Autodesk Inventor part; units mm, degrees
ref_plane "YZ Plane" through (0, 0, 0) normal (1, 0, 0) x (0, 1, 0)
ref_plane "XZ Plane" through (0, 0, 0) normal (0, 1, 0) x (-1, 0, 0)
ref_plane "XY Plane" through (0, 0, 0) normal (0, 0, 1) x (1, 0, 0)
sketch "Sketch1" plane through (0, 0, 0) normal (0, 0, 1) x (1, 0, 0)
  circle A0 centre (0, 0) radius 20
  circle A1 centre (0, 0) radius 23
  dimension "d0" = 40
  dimension "d1" = 46
extrude "Extrusion1" add sketch "Sketch1" along normal mid plane 330
sketch "Sketch2" plane through (0, 0, 0) normal (1, 0, 0) x (0, 1, 0)
  line L0 (0, 210) -> (0, -210)
  line L1 (-210, 0) -> (210, 0)
  point P0 (0, 0)
  point P1 (0, 110)
  point P2 (0, 0)
  point P3 (0, -110)
  dimension "d4" = 110
  dimension "d5" = 110
hole "Hole1" at (0, 0, 110) at (0, 0, 0) at (0, 0, -110) direction (-1, 0, 0) diameter 4.5 end through all
sketch "Sketch3" plane through (0, 0, 0) normal (1, 0, 0) x (0, 1, 0)
  line L0 (23, -145) -> (7, -145)
  line L1 (7, -145) -> (7, 145)
  line L2 (7, 145) -> (23, 145)
  line L3 (23, 145) -> (23, -145)
  line L4 (23, 165) -> (-23, 165)
  line L5 (-23, -165) -> (23, -165)
  line L6 (0, 297.5) -> (0, -297.5)
  point P0 (0, 0)
  dimension "d13" = 20
  dimension "d14" = 20
  dimension "d15" = 7
extrude "Extrusion2" cut sketch "Sketch3" along normal through all both and the other way through all
fillet "Fillet1" radius 2 4 edges at (20.3219, 7, -145) (-20.3219, 7, -145) (20.3219, 7, 145) (-20.3219, 7, 145)
properties part number "Pancake_Tilt Pipe_3 Lanes" material "PVC-Piping"
Geometry: final body of the model. Coordinates: model frame, mm. A direction names the side the tool comes from. Coordinates: 2 decimals unless noted, no trailing zeros. Order: outer loops, then holes, each group sorted by start corner. A loop starts at its lowest first (then second) coordinate and runs counter-clockwise, first axis right, second up.
Item 1: Contact query for flat-ended pins moving along their axis: P1, Ø10, axis at x = 18, y = -6, coming from the -Z side; P2, Ø2.5, axis at x = 21, z = 0.5, coming from the +Y side; P3, Ø10, axis at y = -12.5, z = 69.5, coming from the +X side; P4, Ø3.5, axis at y = 0, z = 0, coming from the -X side. Output: stop coordinate, or through.
Answer:
P1: stops at z = -165
P2: stops at y = 7
P3: stops at x = 21.74
P4: stops at x = 19.92
Item 2: Section query B-B (z = 17). Output: boundary loops of the cut face in (x, y) (3 decimals).
Answer:
outline: (-21.909, 7) arc R23 ccw (long way) to (21.909, 7) - (18.735, 7) arc R20 cw (long way) to (-18.735, 7) - close
Item 3: Access query for faces 4 (the face through (-4.336, -19.524, 2.31)), 5 (the face through (-1.7, 20.1, 145)). Directions: +Z, -Z, +X, -X, +Y, -Y. A direction counts if a zero-diameter tool reaches every point of the face in a straight line with its end or side. Return the directions, or none.
Answer:
face 4: +Z, -Z
face 5: +X, -X, +Y
Item 4: Section query A-A (x = -9). Output: boundary loops of the cut face in (y, z), then the cut area to 3 significant figures.
Answer:
outline: (-21.17, -165) - (-17.86, -165) - (-17.86, 165) - (-21.17, 165) - close; (17.86, -165) - (21.17, -165) - (21.17, -145) - (17.86, -145) - close; (17.86, 145) - (21.17, 145) - (21.17, 165) - (17.86, 165) - close
area: 1,220 mm2
Item 5: Material intervals for line 1 along Z through (x, y) = (18, 13.5); line 2 along X through (y, z) = (0, -29); line 3 along X through (y, z) = (-16, 117), sorted ascending.
Answer:
line 1: z = -165 to -145, 145 to 165
line 2: x = -23 to -20, 20 to 23
line 3: x = -16.52 to -12, 12 to 16.52
Item 6: Draft query along Z for faces 1 (the face through (-1.7, 20.2, -145)), 2 (the face through (-7, 19, 165)), 3 (the face through (-7, 19, -165)). Return one class per face: released by +Z, released by -Z, zero draft, split by the parting line, or undercut.
Answer:
face 1: undercut
face 2: released by +Z
face 3: released by -Z
